Design review of the part built by this model. Coordinates are the model's own, in mm. Give positions to 0.01 mm unless a question says otherwise; leave off trailing zeros. Write each loop counter-clockwise with the first axis right and the second up, starting at its lowest first coordinate (ties: lowest second). Pieces come first, ordered by that corner, then holes. Notation, with made-up numbers: (70.5, 14) -> (118.5, 14) arc R16 ccw to (118.5, 23) -> close; hole circle Ø4 at (14.25, 28). An arc over 180 degrees is marked (long way). Write each question's results on one line, items separated by ' | '. Start each with the question number.
(1) Take a section at C-C (z = 1.7). State the section outline as (x, y) points.
(2) Mouldability with a two-part tool opening along Z and no side actions: class faces 1 (the face through (0.631, 2.514, 2.003)), 2 (the face through (0, 3, -2.3)), 3 (the face through (0, 3, 2.3)) as released by +Z, released by -Z, zero draft, split by the parting line, or undercut.
(3) Take a section at A-A (x = 0). State the section outline as (y, z) points, plus the area to 3 significant figures.
(4) Clearance check with flat-ended pins moving along their axes: pin 1 (1.5 mm diameter, centred on y = 1, z = 1, fed in from -X); pin 2 (2.5 mm diameter, centred on x = 0, z = 0, fed in from -Y). State where each tip first meets the part, or that it passes through.
(5) To check wall thickness, follow probe 1 along X at (y, z) = (4.3, 0.15); probe 2 along Z at (x, y) = (-1.35, 3.05); probe 3 along X at (y, z) = (0.8, -0.55). State the ranges of each line that lie inside material, in increasing order.
(6) Take a section at B-B (y = 4.3). State the section outline as (x, z) points, plus the area to 3 significant figures.
from build123d import *

# Parameters (mm, degrees)
SKETCH1_R           = 3.575
SKETCH1_R_2         = 2.1
BOSS_EXTRUDE1_DEPTH = 5.1
CUT_EXTRUDE1_START  = -10
SKETCH2_R           = 3.575
CUT_EXTRUDE1_DEPTH  = 10


with BuildPart() as part:
    # Sketch1 → Boss-Extrude1 (new body)
    with BuildSketch(Plane(origin=(0, 0, 0), x_dir=(1, 0, 0), z_dir=(0, 1, 0))):
        with Locations(Location((0, 0, 0), (0, 0, 270))):
            Circle(SKETCH1_R)
        with Locations(Location((0, 0, 0), (0, 0, 270))):
            Circle(SKETCH1_R_2, mode=Mode.SUBTRACT)
    extrude(amount=BOSS_EXTRUDE1_DEPTH)

    # Sketch2 → Cut-Extrude1 (cut)
    with BuildSketch(Plane(origin=(0, 5.1, 0), x_dir=(1, 0, 0), z_dir=(0, 1, 0)).offset(CUT_EXTRUDE1_START)):
        Circle(SKETCH2_R)
        Polygon((1.327905619, 2.3), (-1.327905619, 2.3), (-2.655811238, 0), (-1.327905619, -2.3), (1.327905619, -2.3), (2.655811238, 0), align=None, mode=Mode.SUBTRACT)
    extrude(amount=CUT_EXTRUDE1_DEPTH, mode=Mode.SUBTRACT)


solid = part.part
Report:
1) outline: (-1.67, 0) -> (-1.23, 0) -> (-1.23, 5.1) -> (-1.67, 5.1) -> close; (1.23, 0) -> (1.67, 0) -> (1.67, 5.1) -> (1.23, 5.1) -> close
2) face 1: undercut | face 2: released by -Z | face 3: released by +Z
3) outline: (0, -2.3) -> (5.1, -2.3) -> (5.1, -2.1) -> (0, -2.1) -> close; (0, 2.1) -> (5.1, 2.1) -> (5.1, 2.3) -> (0, 2.3) -> close | area: 2.04 mm2
4) pin 1: x = -2.51 | pin 2: through
5) probe 1: -2.57 to -2.09, 2.09 to 2.57 | probe 2: -2.26 to -1.61, 1.61 to 2.26 | probe 3: -2.34 to -2.03, 2.03 to 2.34
6) outline: (-2.66, 0) -> (-1.33, -2.3) -> (1.33, -2.3) -> (2.66, 0) -> (1.33, 2.3) -> (-1.33, 2.3) -> close; hole circle Ø4.2 at (0, 0) | area: 4.47 mm2
